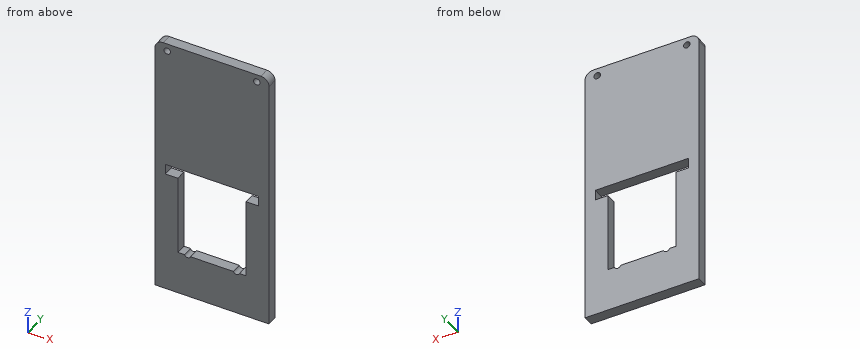
from build123d import *

# Parameters (mm, degrees)
BOSS_EXTRUDE1_DEPTH = 3.175
CUT_EXTRUDE1_DEPTH  = 204.138678001
SKETCH3_W           = 42
SKETCH3_H           = 55.35
SKETCH3_W_2         = 7.65
SKETCH3_H_2         = 6.35
CUT_EXTRUDE2_DEPTH  = 204.138678001
FILLET3_R           = 5
SKETCH5_R           = 2
CUT_EXTRUDE4_DEPTH  = 204.138678001


with BuildPart() as part:
    # Sketch1 → Boss-Extrude1 (new, symmetric)
    with BuildSketch(Plane(origin=(0, 0, 0), x_dir=(1, 0, 0), z_dir=(0, 1, 0))):
        with BuildLine():
            Line((35, -200), (35, 0))
            ThreePointArc((35, 0), (0, 35), (-35, 0))
            Line((-35, 0), (-35, -200))
            Line((-35, -200), (35, -200))
        make_face()
    extrude(amount=BOSS_EXTRUDE1_DEPTH, both=True)

    # Sketch2 → Cut-Extrude1 (cut, through all)
    with BuildSketch(Plane(origin=(0, 3.175, 0), x_dir=(1, 0, 0), z_dir=(0, 1, 0))):
        with BuildLine():
            Line((-35, -38), (35, -38))
            Line((35, -38), (35, 0))
            ThreePointArc((35, 0), (0, 35), (-35, 0))
            Line((-35, 0), (-35, -38))
        make_face()
    extrude(amount=-CUT_EXTRUDE1_DEPTH, mode=Mode.SUBTRACT)

    # Sketch3 → Cut-Extrude2 (cut, through all)
    with BuildSketch(Plane(origin=(0, 3.175, 0), x_dir=(1, 0, 0), z_dir=(0, 1, 0))):
        with Locations((0, -92.325)):
            Rectangle(SKETCH3_W, SKETCH3_H)
        with Locations((-24.825, -116.825)):
            Rectangle(SKETCH3_W_2, SKETCH3_H_2)
        with Locations((24.825, -116.825)):
            Rectangle(SKETCH3_W_2, SKETCH3_H_2)
    extrude(amount=-CUT_EXTRUDE2_DEPTH, mode=Mode.SUBTRACT)

    # Fillet3
    fillet3_edges = [part.edges().sort_by_distance(p)[0] for p in [
        (35, 0, 200),
        (-35, 0, 200),
    ]]
    fillet(fillet3_edges, radius=FILLET3_R)

    # Sketch5 → Cut-Extrude4 (cut, through all)
    with BuildSketch(Plane(origin=(0, 3.175, 0), x_dir=(1, 0, 0), z_dir=(0, 1, 0))):
        with Locations(Location((27.5, -195.35, 0), (0, 0, 270))):
            Circle(SKETCH5_R)
        with Locations(Location((-27.5, -195.35, 0), (0, 0, 270))):
            Circle(SKETCH5_R)
        with Locations((15, -65.35)):
            Circle(SKETCH5_R)
        with Locations((-15, -65.35)):
            Circle(SKETCH5_R)
    extrude(amount=-CUT_EXTRUDE4_DEPTH, mode=Mode.SUBTRACT)


solid = part.part
Can you work these out from the model? Positions are in its coordinate system, mm. Coordinates: 2 decimals unless noted, no trailing zeros. Write each loop counter-clockwise with the first axis right and the second up, starting at its lowest first coordinate (ties: lowest second). Pieces come first, ordered by that corner, then holes. Notation, with made-up numbers: M 15.5,82.25 L 28.5,82.25 A15 ccw 28.5,91.25 Z; hole C 66,72.5 d1. An arc over 180 degrees is marked long. Use one line per item in the form item = value.
Q1. I need wall thicknesses on line 1 along X through (y, z) = (1.25, 195.35); line 2 along X through (y, z) = (-0.75, 93.5); line 3 along X through (y, z) = (2.5, 119). Which ranges of each line are inside material? Lowest first, please. Write a range as from..to.
Model answer:
line_1 = -34.99..-29.5, -25.5..25.5, 29.5..34.99
line_2 = -35..-21, 21..35
line_3 = -35..-28.65, 28.65..35
Q2. If we section it at C-C (y = -1.5): Write out the boundary of the cut face in (x, z).
Model answer:
outline = M -35,38 L 35,38 L 35,195 A5 ccw 30,200 L -30,200 A5 ccw -35,195 Z; hole C -27.5,195.35 d4; hole M -28.65,113.65 L -21,113.65 L -21,64.65 L -16.87,64.65 A2 ccw -13.13,64.65 L 13.13,64.65 A2 ccw 16.87,64.65 L 21,64.65 L 21,113.65 L 28.65,113.65 L 28.65,120 L -28.65,120 Z; hole C 27.5,195.35 d4
Q3. If we section it at B-B (x = -23.5): Write out the boundary of the cut face in (y, z) (3 decimals), then the cut area to 3 significant figures.
Model answer:
outline = M -3.175,38 L 3.175,38 L 3.175,113.65 L -3.175,113.65 Z; M -3.175,120 L 3.175,120 L 3.175,200 L -3.175,200 Z
area = 988 mm^2
Q4. For P1, Ø4.5, axis at x = 27.5, z = 195.35, coming from the +Y side (3 decimals), with a flat end and sliding along its axis, tell me the tip position at first contact or that it passes through.
Model answer:
P1 = 3.175
Q5. If we section it at A-A (z = 78.5): Write out the boundary of the cut face in (x, y) (3 decimals), then the cut area to 3 significant figures.
Model answer:
outline = M -35,-3.175 L -21,-3.175 L -21,3.175 L -35,3.175 Z; M 21,-3.175 L 35,-3.175 L 35,3.175 L 21,3.175 Z
area = 178 mm^2
